Job drawing, mm, ordinate dimensions from the low corner. One solid piece. Round coordinates to 2 decimals unless told otherwise and drop trailing zeros. Loops run counter-clockwise (first coordinate to the right, second up) from the corner with the lowest first, then second, coordinate; pieces in that order, holes last.
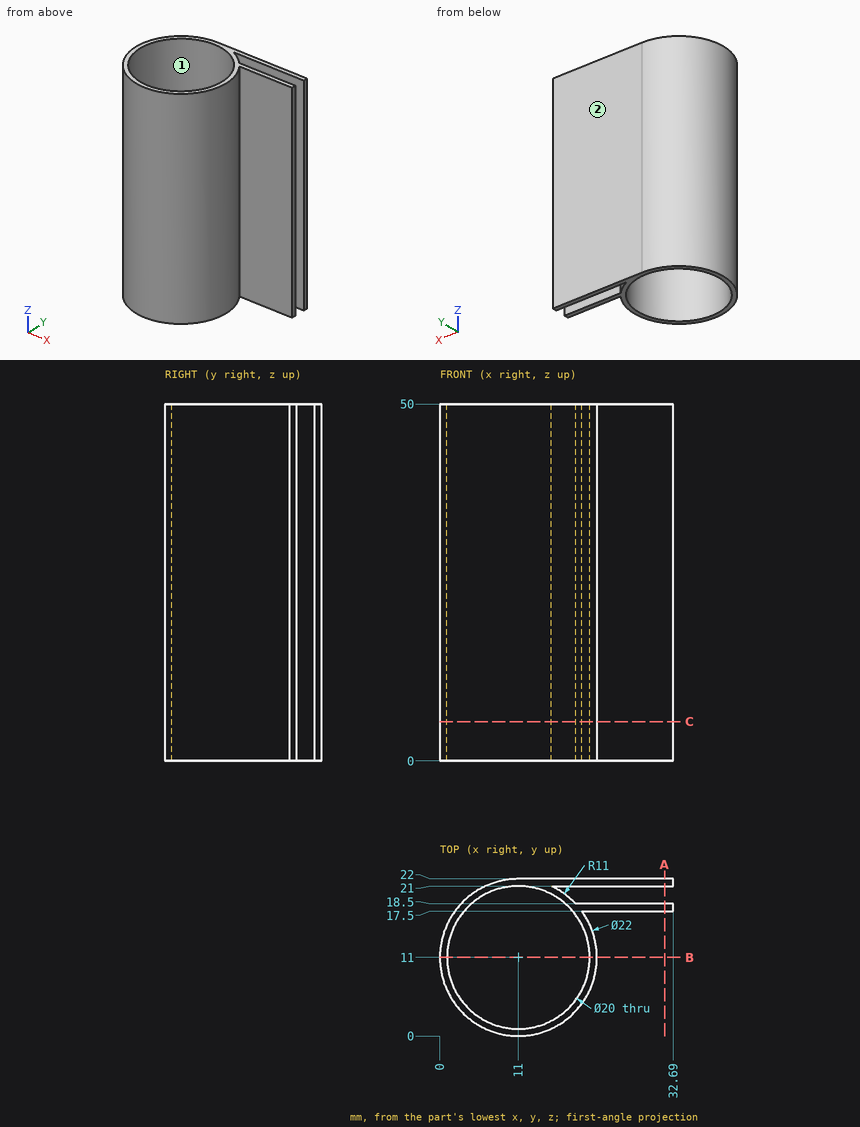
(1) Slice it at A-A on x = 31.5. List the corners of the cut face in (y, z).
Responses:
outline: (17.5, 0) - (18.5, 0) - (18.5, 50) - (17.5, 50) - close; (21, 0) - (22, 0) - (22, 50) - (21, 50) - close
(2) Pin check, flat tips, straight feed: P1, Ø12, axis at x = 23, z = 5.5, coming from the -Y side; P2, Ø12, axis at y = 6, z = 11, coming from the -X side; P3, Ø19, axis at x = 24, z = 28.5, coming from the -Y side; P4, Ø2, axis at y = 12.5, z = 19.5, coming from the +X side. Stop position of each tip, or through.
Responses:
P1: stops at y = 1.78
P2: stops at x = 0
P3: stops at y = 0.57
P4: stops at x = 21.99
(3) Slice it at C-C on z = 5.5. List the corners of the cut face in (x, y).
Responses:
outline: (11, 22) arc R11 ccw (long way) to (19.87, 17.5) - (32.69, 17.5) - (32.69, 18.5) - (19.05, 18.5) arc R11 ccw to (15.58, 21) - (32.69, 21) - (32.69, 22) - close; hole circle Ø20 at (11, 11)
(4) Slice it at B-B on y = 11. List the corners of the cut face in (x, z), plus the area to 3 significant figures.
Responses:
outline: (0, 0) - (1, 0) - (1, 50) - (0, 50) - close; (21, 0) - (22, 0) - (22, 50) - (21, 50) - close
area: 100 mm2
(5) Pull direction Y, two halves, no side cores. Call the marked faces 1 and 2: +Y half, -Y half, draft (parallel to the pull), parting line (faces both ways), or undercut.
Responses:
face 1: undercut
face 2: +Y half
(6) Probe line 1 (Y direction, x = 31, z = 15); line 2 (Y direction, x = 19, z = 10); line 3 (Y direction, x = 10.5, z = 27). List the from-to ranges inside material, lowest first.
Responses:
line 1: y = 17.5 to 18.5, 21 to 22
line 2: y = 3.45 to 5, 17 to 18.55, 21 to 22
line 3: y = 0.01 to 1.01, 20.99 to 21.99
